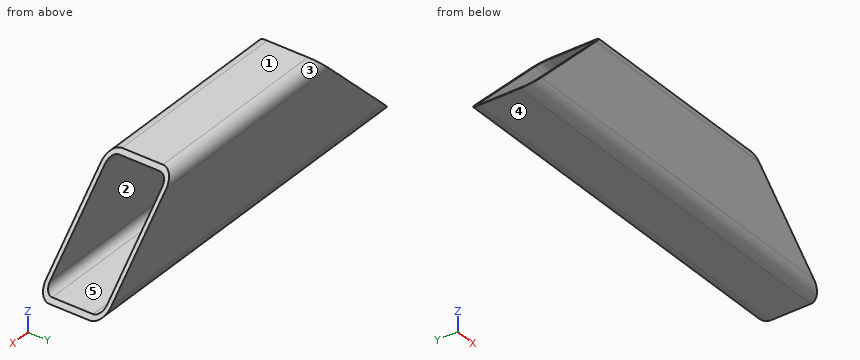
Autodesk Inventor part; units mm, degrees
ref_plane "YZ Plane" through (0, 0, 0) normal (1, 0, 0) x (0, 1, 0)
ref_plane "XZ Plane" through (0, 0, 0) normal (0, 1, 0) x (-1, 0, 0)
ref_plane "XY Plane" through (0, 0, 0) normal (0, 0, 1) x (1, 0, 0)
sketch "Sketch1" plane through (0, 0, 0) normal (1, 0, 0) x (0, 1, 0)
  line L0 (-15.875, 38.1) -> (15.875, 38.1)
  line L1 (25.4, 28.575) -> (25.4, -28.575)
  line L2 (15.875, -38.1) -> (-15.875, -38.1)
  line L3 (-25.4, -28.575) -> (-25.4, 28.575)
  line L4 (-25.4, 38.1) -> (25.4, -38.1) construction
  line L5 (25.4, 38.1) -> (-25.4, -38.1) construction
  arc A0 (25.4, 28.575) -> (15.875, 38.1) centre (15.875, 28.575) ccw
  arc A1 (-15.875, 38.1) -> (-25.4, 28.575) centre (-15.875, 28.575) ccw
  arc A2 (-25.4, -28.575) -> (-15.875, -38.1) centre (-15.875, -28.575) ccw
  arc A3 (15.875, -38.1) -> (25.4, -28.575) centre (15.875, -28.575) ccw
  line L6 (22.225, -28.575) -> (22.225, 28.575)
  arc A4 (22.225, 28.575) -> (15.875, 34.925) centre (15.875, 28.575) ccw
  line L7 (15.875, 34.925) -> (-15.875, 34.925)
  arc A5 (-15.875, 34.925) -> (-22.225, 28.575) centre (-15.875, 28.575) ccw
  line L8 (-22.225, 28.575) -> (-22.225, -28.575)
  arc A6 (-22.225, -28.575) -> (-15.875, -34.925) centre (-15.875, -28.575) ccw
  line L9 (-15.875, -34.925) -> (15.875, -34.925)
  arc A7 (15.875, -34.925) -> (22.225, -28.575) centre (15.875, -28.575) ccw
  point P0 (0, 0)
  dimension "d0" = 76.2
  dimension "d1" = 50.8
  dimension "d2" = 9.525
  dimension "d3" = 3.175
extrude "Extrusion1" add sketch "Sketch1" along normal mid plane 303.8
sketch "Sketch2" plane through (-151.9, 25.4, 28.575) normal (0, 1, 0) x (1, 0, 0)
  line L0 (303.8, 57.15) -> (303.8, 66.675)
  line L1 (303.8, 66.675) -> (227.6, -9.525)
  line L2 (0, -9.525) -> (303.8, -9.525)
  line L3 (303.8, 66.675) -> (411.5631, 66.675) construction
  line L4 (227.6, -9.525) -> (303.8, -9.525)
  line L5 (303.8, -9.525) -> (303.8, 66.675)
  line L6 (151.9, 28.575) -> (151.9, -9.525)
  line L7 (0, 66.675) -> (76.2, -9.525)
  line L8 (76.2, -9.525) -> (0, -9.525)
  line L9 (0, -9.525) -> (0, 66.675)
  dimension "d6" = 135
extrude "Extrusion2" cut sketch "Sketch2" against normal through all
equation "\"d0\" = stockWidth"
equation "\"d1\" = stockHeight"
equation "\"d2\" = stockRad"
equation "\"d3\" = stockGuage"
equation "\"height\" = 203.2"
equation "\"shaftDiam\" = 6.35"
equation "\"shaftSpace\" = 1.5875"
equation "\"stageSpace\" = 2.54"
equation "\"stageAngle\" = 15deg"
equation "\"stockHeight\" = 50.8"
equation "\"stockWidth\" = 76.2"
equation "\"stockRad\" = 9.525"
equation "\"stockGuage\" = 3.175"
equation "\"groundActu\" = 304.8"
equation "\"baseWidth\" = 1066.8"
equation "\"baseDepth\" = 254"
equation "\"capThickness\" = 3.175"
equation "\"sup1Ang\" = 22.619865deg"
equation "\"sup1Len\" = 660.4"
equation "\"supVertLen\" = 955.13561"
equation "\"sup2Ang\" = 8.959949deg"
equation "\"sup2Len\" = 2079.37366"
equation "\"supSideAng\" = 19.376933deg"
equation "\"supSideLen\" = 1531.12879"
equation "\"FlangeDiam\" = 12.7"
equation "\"bearingDiam\" = 9.5504"
equation "\"FlangeDepth\" = 1.5875"
equation "\"smallFilet\" = 0.39687"
equation "\"thickness\" = 12.7"
equation "\"ringDiam\" = 96.46608"
properties part number "back bar" material "Aluminum 6061"
Input: part model. Units: mm. Frame: model coordinates. Face numbers are marked on the shaded views. A direction names the side the tool comes from. Round coordinates to 2 decimals unless told otherwise and drop trailing zeros. Order: outer loops, then holes, each group sorted by start corner. A loop starts at its lowest first (then second) coordinate and runs counter-clockwise, first axis right, second up. Notation, with made-up numbers: (71, -27.5) - (122, -27.5) arc R16 cw to (122, -0.5) - close; hole circle Ø4 at (24.25, -25). An arc over 180 degrees is marked (long way). Answer in a Markdown table with one row per item.
Item 1: Section query B-B (y = -5). Return the cut outline in (x, z) (3 decimals).
Model answer:
| item | result |
|---|---|
| outline | (-151.9, -38.1) - (151.9, -38.1) - (148.725, -34.925) - (-148.725, -34.925) - close; (-78.875, 34.925) - (78.875, 34.925) - (75.7, 38.1) - (-75.7, 38.1) - close |
Item 2: Mould query, pull axis Y, two halves, no side actions, for the marked faces 3, 4 and 5. Classes: released by +Y, released by -Y, zero draft, split by the parting line, or undercut.
Model answer:
| item | result |
|---|---|
| face 3 | released by +Y |
| face 4 | zero draft |
| face 5 | undercut |
Item 3: Pin query (flat end, axial travel): pin 1 (5 mm diameter, centred on x = -95, y = -5.5, fed in from +Z) (3 decimals); pin 2 (8 mm diameter, centred on y = -16, z = 26.5, fed in from -X). Return the tip coordinate at first contact, or that it passes through.
Model answer:
| item | result |
|---|---|
| pin 1 | stops at z = -34.925 |
| pin 2 | passes through |
Item 4: Reachability of the marked faces 1 and 2 from +Z, -Z, +X, -X, +Y, -Y: full face, straight path, thin tool, end or side. Return the list, or none.
Model answer:
| item | result |
|---|---|
| face 1 | +Z, +X, -X, +Y, -Y |
| face 2 | +X, -X |
Item 5: Section query A-A (z = -8). Return the cut outline in (x, y) (3 decimals), then the cut area to 3 significant figures.
Model answer:
| item | result |
|---|---|
| outline | (-121.8, -25.4) - (121.8, -25.4) - (121.8, -22.225) - (-121.8, -22.225) - close; (-121.8, 22.225) - (121.8, 22.225) - (121.8, 25.4) - (-121.8, 25.4) - close |
| area | 1,550 mm² |
Item 6: Line query: line 1 (Y direction, x = 27.5, z = 14) (3 decimals); line 2 (Z direction, x = 25.5, y = 11) (3 decimals); line 3 (Z direction, x = -132.5, y = -0.5) (3 decimals). Output: solid intervals per line, ascending.
Model answer:
| item | result |
|---|---|
| line 1 | y = -25.4 to -22.225, 22.225 to 25.4 |
| line 2 | z = -38.1 to -34.925, 34.925 to 38.1 |
| line 3 | z = -38.1 to -34.925 |
Item 7: Section query C-C (x = 16). Return the cut outline in (y, z) (3 decimals).
Model answer:
| item | result |
|---|---|
| outline | (-25.4, -28.575) arc R9.525 ccw to (-15.875, -38.1) - (15.875, -38.1) arc R9.525 ccw to (25.4, -28.575) - (25.4, 28.575) arc R9.525 ccw to (15.875, 38.1) - (-15.875, 38.1) arc R9.525 ccw to (-25.4, 28.575) - close; hole (-22.225, -28.575) arc R6.35 ccw to (-15.875, -34.925) - (15.875, -34.925) arc R6.35 ccw to (22.225, -28.575) - (22.225, 28.575) arc R6.35 ccw to (15.875, 34.925) - (-15.875, 34.925) arc R6.35 ccw to (-22.225, 28.575) - close |
Item 8: Section query D-D (x = 125). Return the cut outline in (y, z) (3 decimals), then the cut area to 3 significant figures.
Model answer:
| item | result |
|---|---|
| outline | (-25.4, -28.575) arc R9.525 ccw to (-15.875, -38.1) - (15.875, -38.1) arc R9.525 ccw to (25.4, -28.575) - (25.4, -11.2) - (22.225, -11.2) - (22.225, -28.575) arc R6.35 cw to (15.875, -34.925) - (-15.875, -34.925) arc R6.35 cw to (-22.225, -28.575) - (-22.225, -11.2) - (-25.4, -11.2) - close |
| area | 290 mm² |
